Source: three-view drawing plus pictorial views. Frame: mm from the lowest corner of the part. Give positions to 0.01 mm unless a question says otherwise; leave off trailing zeros. Write each loop counter-clockwise with the first axis right and the second up, starting at its lowest first coordinate (ties: lowest second). Pieces come first, ordered by that corner, then holes.
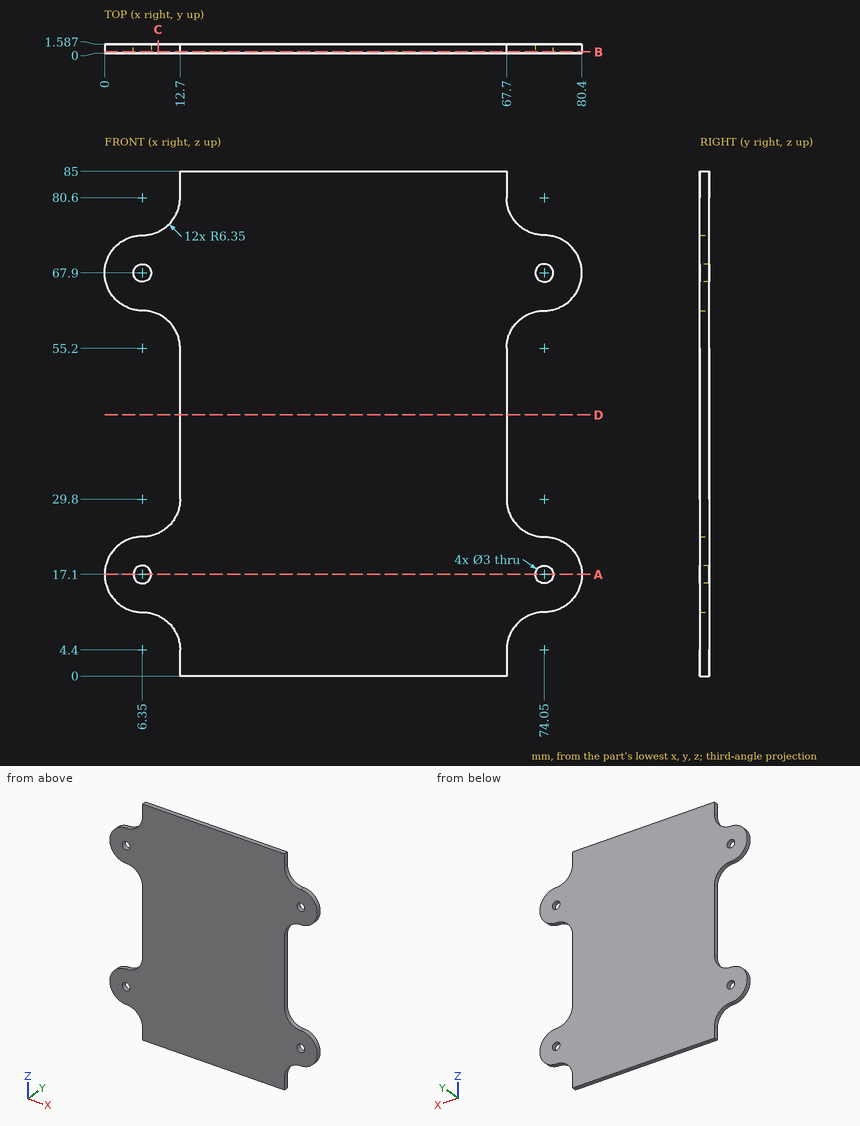
Q1. Pin query (flat end, axial travel): P1, Ø1.8, axis at x = 6.35, z = 67.9, coming from the -Y side; P2, Ø0.5, axis at y = 0.5, z = 48.5, coming from the -X side; P3, Ø0.8, axis at y = 0.5, z = 82.5, coming from the +X side. Return the tip coordinate at first contact, or that it passes through.
Filled sheet:
P1: passes through
P2: stops at x = 12.7
P3: stops at x = 67.7
Q2. Ray query, line 1 along X through (y, z) = (0.85, 67.9); line 2 along Z through (x, y) = (6.5, 1.4); line 3 along X through (y, z) = (0.4, 31). Return the intervals inside material, ascending.
Filled sheet:
line 1: x = 0 to 4.85, 7.85 to 72.55, 75.55 to 80.4
line 2: z = 10.75 to 15.61, 18.59 to 23.45, 61.55 to 66.41, 69.39 to 74.25
line 3: x = 12.7 to 67.7
Q3. Section A-A on z = 17.1. Output: boundary loops of the cut face in (x, y), plus the area to 3 significant figures.
Filled sheet:
outline: (0, 0) - (4.85, 0) - (4.85, 1.59) - (0, 1.59) - close; (7.85, 0) - (72.55, 0) - (72.55, 1.59) - (7.85, 1.59) - close; (75.55, 0) - (80.4, 0) - (80.4, 1.59) - (75.55, 1.59) - close
area: 118 mm2
Q4. Section D-D on z = 44. Output: boundary loops of the cut face in (x, y).
Filled sheet:
outline: (12.7, 0) - (67.7, 0) - (67.7, 1.59) - (12.7, 1.59) - close
Q5. Section B-B on y = 0.25. Output: boundary loops of the cut face in (x, z), plus the area to 3 significant figures.
Filled sheet:
outline: (6.35, 10.75) arc R6.35 cw to (12.7, 4.4) - (12.7, 0) - (67.7, 0) - (67.7, 4.4) arc R6.35 cw to (74.05, 10.75) arc R6.35 ccw to (74.05, 23.45) arc R6.35 cw to (67.7, 29.8) - (67.7, 55.2) arc R6.35 cw to (74.05, 61.55) arc R6.35 ccw to (74.05, 74.25) arc R6.35 cw to (67.7, 80.6) - (67.7, 85) - (12.7, 85) - (12.7, 80.6) arc R6.35 cw to (6.35, 74.25) arc R6.35 ccw to (6.35, 61.55) arc R6.35 cw to (12.7, 55.2) - (12.7, 29.8) arc R6.35 cw to (6.35, 23.45) arc R6.35 ccw to start; hole circle Ø3 at (6.35, 17.1); hole circle Ø3 at (6.35, 67.9); hole circle Ø3 at (74.05, 17.1); hole circle Ø3 at (74.05, 67.9)
area: 5,290 mm2
Q6. Section C-C on x = 9. Output: boundary loops of the cut face in (y, z).
Filled sheet:
outline: (0, 10.17) - (1.59, 10.17) - (1.59, 24.03) - (0, 24.03) - close; (0, 60.97) - (1.59, 60.97) - (1.59, 74.83) - (0, 74.83) - close
